Geometry: see drawing. Coordinates: mm, zero at the bounding-box minimum. A direction names the side the tool comes from. Round coordinates to 2 decimals unless told otherwise and drop trailing zeros. Write each loop counter-clockwise with the first axis right and the second up, starting at its lowest first coordinate (ties: lowest second). Pieces come first, ordered by that corner, then holes. Notation, with made-up numbers: M 43.5,69 L 77.5,69 A25 cw 77.5,97 Z; hole C 52.5,-36.75 d5. An arc over 180 degrees is marked long. Use a Markdown table: item, result.
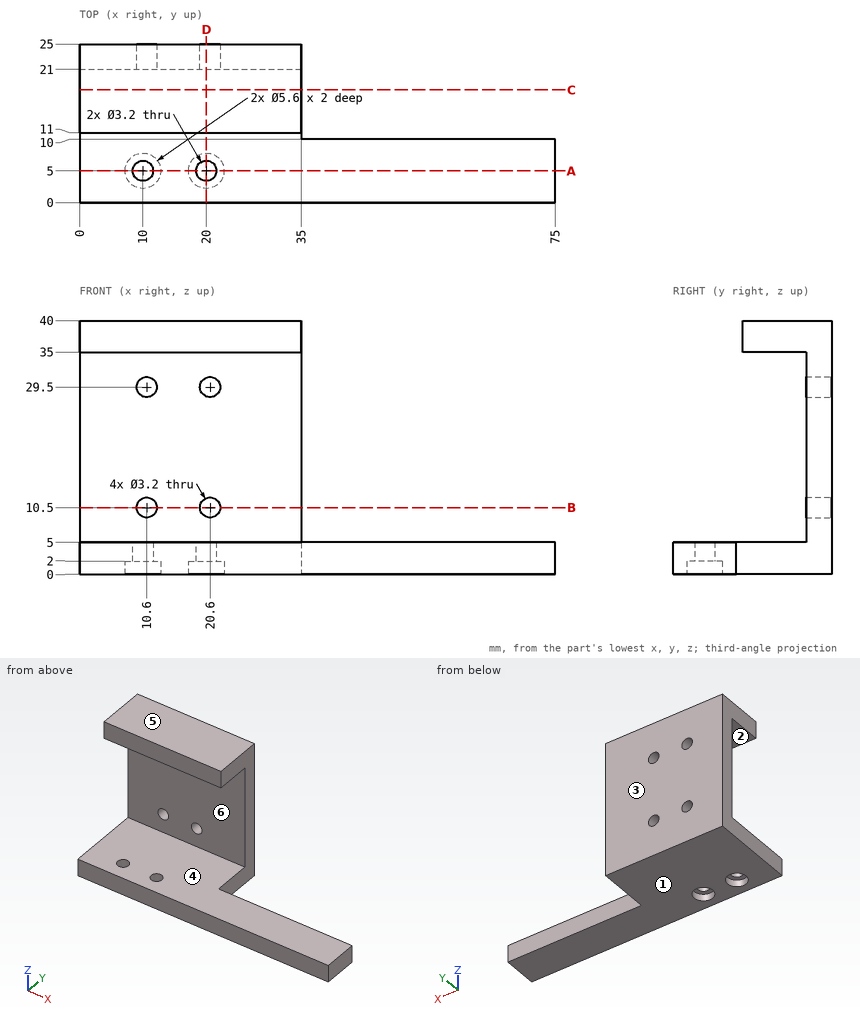
Q1. Reachability of the marked faces 5 and 6 from +Z, -Z, +X, -X, +Y, -Y: full face, straight path, thin tool, end or side. Return the list, or none.
Results are:
| item | result |
|---|---|
| face 5 | +Z, +X, -X, +Y, -Y |
| face 6 | +X, -X, -Y |
Q2. Section D-D on x = 20. Return loops of the section in (y, z).
Results are:
| item | result |
|---|---|
| outline | M 0,0 L 2.2,0 L 2.2,2 L 3.4,2 L 3.4,5 L 0,5 Z; M 6.6,2 L 7.8,2 L 7.8,0 L 25,0 L 25,9.02 L 21,9.02 L 21,5 L 6.6,5 Z; M 11,35 L 21,35 L 21,30.98 L 25,30.98 L 25,40 L 11,40 Z; M 21,11.98 L 25,11.98 L 25,28.02 L 21,28.02 Z |
Q3. Mould query, pull axis Z, two halves, no side actions, for the marked faces 1, 2, 3 and 4. Classes: +Z half, -Z half, draft (parallel to the pull), parting line (faces both ways), or undercut.
Results are:
| item | result |
|---|---|
| face 1 | -Z half |
| face 2 | undercut |
| face 3 | draft |
| face 4 | undercut |
Q4. First-contact query: pin 1 Ø5 at (x, z) = (35.5, 32) entering from -Y; pin 2 Ø5 at (x, y) = (20, 21.5) entering from -Z; pin 3 Ø12 at (y, z) = (19.5, 21) entering from +X; pin 4 Ø4.5 at (x, y) = (20, 4.5) entering from -Z. Flat tips, straight axial feed; report the tip coordinate or a pass-through.
Results are:
| item | result |
|---|---|
| pin 1 | y = 21 |
| pin 2 | z = 0 |
| pin 3 | x = 35 |
| pin 4 | z = 2 |
Q5. Section B-B on z = 10.5. Return loops of the section in (x, y), plus the area to 3 significant figures.
Results are:
| item | result |
|---|---|
| outline | M 0,21 L 9,21 L 9,25 L 0,25 Z; M 12.2,21 L 19,21 L 19,25 L 12.2,25 Z; M 22.2,21 L 35,21 L 35,25 L 22.2,25 Z |
| area | 114 mm^2 |
Q6. Section A-A on y = 5. Return loops of the section in (x, z).
Results are:
| item | result |
|---|---|
| outline | M 0,0 L 7.2,0 L 7.2,2 L 8.4,2 L 8.4,5 L 0,5 Z; M 11.6,2 L 12.8,2 L 12.8,0 L 17.2,0 L 17.2,2 L 18.4,2 L 18.4,5 L 11.6,5 Z; M 21.6,2 L 22.8,2 L 22.8,0 L 75,0 L 75,5 L 21.6,5 Z |
Q7. Line query: L1, parallel to X at y = 22.3, z = 29.5; L2, parallel to Z at x = 20.6, y = 23.75; L3, parallel to Z at x = 4, y = 11.75. Output: solid intervals per line, ascending.
Results are:
| item | result |
|---|---|
| L1 | 0 to 9, 12.2 to 19, 22.2 to 35 |
| L2 | 0 to 8.9, 12.1 to 27.9, 31.1 to 40 |
| L3 | 0 to 5, 35 to 40 |
Q8. Section C-C on y = 17.75. Return loops of the section in (x, z).
Results are:
| item | result |
|---|---|
| outline | M 0,0 L 35,0 L 35,5 L 0,5 Z; M 0,35 L 35,35 L 35,40 L 0,40 Z |
